Geometry check sheet. Reference: the model listing, model coordinates, mm. A direction names the side the tool comes from. Give positions to 0.01 mm unless a question says otherwise; leave off trailing zeros. Write each loop counter-clockwise with the first axis right and the second up, starting at its lowest first coordinate (ties: lowest second). Pieces come first, ordered by that corner, then holes. Notation, with made-up numbers: (1, 43.25) - (15, 43.25) arc R10 cw to (15, 61.25) - close; hole circle Ø10 at (-30, -19). An arc over 180 degrees is marked (long way). Use a Markdown table: item, result.
```python
from build123d import *

# Parameters (mm, degrees)
SKETCH2_W           = 155
SKETCH2_H           = 80
SKETCH2_R           = 1
BOSS_EXTRUDE1_DEPTH = 5
SKETCH3_W           = 155
SKETCH3_H           = 80
SKETCH3_W_2         = 149
SKETCH3_H_2         = 74
BOSS_EXTRUDE2_DEPTH = 10
SKETCH4_W           = 155
SKETCH4_H           = 80
SKETCH4_W_2         = 145
SKETCH4_H_2         = 70
BOSS_EXTRUDE3_DEPTH = 7
FILLET1_R           = 2


with BuildPart() as part:
    # Sketch2 → Boss-Extrude1 (new body)
    with BuildSketch(Plane(origin=(0, 0, 0), x_dir=(1, 0, 0), z_dir=(0, 1, 0))):
        with Locations((77.5, 40)):
            Rectangle(SKETCH2_W, SKETCH2_H)
        with Locations(Location((40, 40, 0), (0, 0, 270))):  # turned: the seam where the file's is
            Circle(SKETCH2_R, mode=Mode.SUBTRACT)
        with Locations(Location((115, 40, 0), (0, 0, 270))):  # turned: the seam where the file's is
            Circle(SKETCH2_R, mode=Mode.SUBTRACT)
        with Locations(Location((73, 65, 0), (0, 0, 270))):  # turned: the seam where the file's is
            Circle(SKETCH2_R, mode=Mode.SUBTRACT)
        with Locations(Location((73, 15, 0), (0, 0, 270))):  # turned: the seam where the file's is
            Circle(SKETCH2_R, mode=Mode.SUBTRACT)
    extrude(amount=-BOSS_EXTRUDE1_DEPTH)

    # Sketch3 → Boss-Extrude2 (add)
    with BuildSketch(Plane(origin=(0, 0, 0), x_dir=(1, 0, 0), z_dir=(0, 1, 0))):
        with Locations((77.5, 40)):
            Rectangle(SKETCH3_W, SKETCH3_H)
        with Locations((77.5, 40)):
            Rectangle(SKETCH3_W_2, SKETCH3_H_2, mode=Mode.SUBTRACT)
    extrude(amount=-BOSS_EXTRUDE2_DEPTH)

    # Sketch4 → Boss-Extrude3 (add)
    with BuildSketch(Plane(origin=(0, 0, 0), x_dir=(1, 0, 0), z_dir=(0, 1, 0))):
        with Locations((77.5, 40)):
            Rectangle(SKETCH4_W, SKETCH4_H)
        with Locations((77.5, 40)):
            Rectangle(SKETCH4_W_2, SKETCH4_H_2, mode=Mode.SUBTRACT)
    extrude(amount=-BOSS_EXTRUDE3_DEPTH)

    # Fillet1
    fillet1_edges = [part.edges().sort_by_distance(p)[0] for p in [
        (77.5, 0, -80),
        (155, 0, -40),
        (77.5, 0, 0),
        (0, 0, -40),
        (0, -5, -80),
        (155, -5, -80),
        (155, -5, 0),
        (0, -5, 0),
    ]]
    fillet(fillet1_edges, radius=FILLET1_R)


solid = part.part
```
1) Set-up check for faces 1 (the flat face through (54, -10, -79)), 2 (the flat face through (76, -8, -77)): record each of +Z, -Z, +X, -X, +Y, -Y from which the full face is reachable in a straight line by a thin tool's end or side.
Working result:
| item | result |
|---|---|
| face 1 | +Z, -Z, +X, -X, -Y |
| face 2 | -Y |
2) Depth check by flat-ended pin: P1, Ø2.5, axis at x = 73, z = -15, coming from the +Y side; P2, Ø22, axis at x = 96, z = -49, coming from the -Y side. Enter the tip coordinate at first touch or a pass-through.
Working result:
| item | result |
|---|---|
| P1 | stops at y = 0 |
| P2 | stops at y = -5 |
3) Section check B-B on x = 49. Record the boundary of the cut face in (y, z).
Working result:
| item | result |
|---|---|
| outline | (-10, -80) - (-2, -80) arc R2 ccw to (0, -78) - (0, -2) arc R2 ccw to (-2, 0) - (-10, 0) - (-10, -3) - (-7, -3) - (-7, -5) - (-5, -5) - (-5, -75) - (-7, -75) - (-7, -77) - (-10, -77) - close |
4) Mould release check, pull along X, two halves, no side actions. Record for faces 3 (the flat face through (0, -6, -39)), 4 (the flat face through (76, -6, 0)), 5 (the flat face through (152, -8, -39)): pulls with the +X half, pulls with the -X half, needs draft (parallel to the pull), parting line crosses it, or undercut.
Working result:
| item | result |
|---|---|
| face 3 | pulls with the -X half |
| face 4 | needs draft |
| face 5 | undercut |
5) Section check A-A on z = -57. Record the boundary of the cut face in (x, y), then the cut area to 3 significant figures.
Working result:
| item | result |
|---|---|
| outline | (0, -10) - (3, -10) - (3, -7) - (5, -7) - (5, -5) - (150, -5) - (150, -7) - (152, -7) - (152, -10) - (155, -10) - (155, -2) arc R2 ccw to (153, 0) - (2, 0) arc R2 ccw to (0, -2) - close |
| area | 811 mm² |
6) Material ranges on L1, parallel to X at y = -3.55, z = -40; L2, parallel to Z at x = 73, y = -1.7; L3, parallel to X at y = -9.25, z = -56, recorded low to high. Write a range as from..to.
Working result:
| item | result |
|---|---|
| L1 | x = 0..39, 41..114, 116..155 |
| L2 | z = -79.98..-66, -64..-16, -14..-0.02 |
| L3 | x = 0..3, 152..155 |
